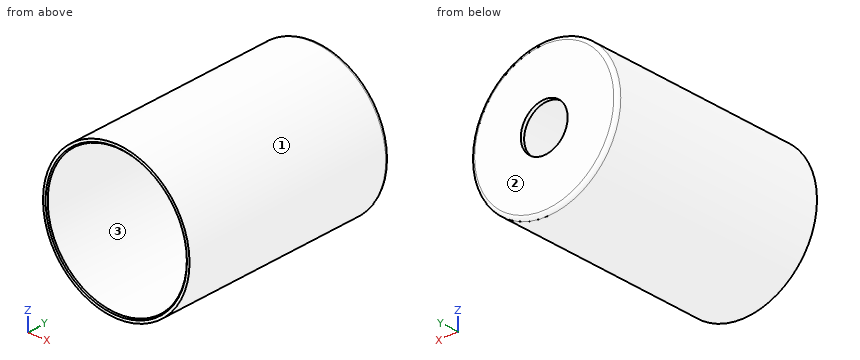
```python
from build123d import *

# Parameters (mm, degrees)
F0_R          = 50.8
F1_DEPTH      = 152.4
F2_T          = -2.54
F3_R          = 16.25
F4_DEPTH      = 25.4
F4_DEPTH_BACK = 25.4
F5_SIZE       = 0.762
F6_R          = 2.54


with BuildPart() as f1:
    # F0 (on Front) → F1 (new body)
    with BuildSketch(Plane.XZ):
        Circle(F0_R)
    extrude(amount=F1_DEPTH)

    # F2
    f2_openings = [f1.faces().sort_by_distance(p)[0] for p in [
        (0, -152.4, 0),
    ]]
    offset(amount=F2_T, openings=f2_openings)

    # F3 (on face) → F4 (cut, two sides)
    with BuildSketch(Plane.XZ.offset(2.54)) as f4_sk:
        Circle(F3_R)
    extrude(amount=-F4_DEPTH, mode=Mode.SUBTRACT)
    extrude(f4_sk.sketch, amount=F4_DEPTH_BACK, mode=Mode.SUBTRACT)

    # F5
    f5_edges = [f1.edges().sort_by_distance(p)[0] for p in [
        (-48.26, -152.4, 0),
    ]]
    chamfer(f5_edges, length=F5_SIZE)

    # F6
    f6_edges = [f1.edges().sort_by_distance(p)[0] for p in [
        (-50.8, 0, 0),
    ]]
    fillet(f6_edges, radius=F6_R)


solid = f1.part
```
Here's how the part is built. I have some questions about the finished solid (model axes, mm). Face numbers are marked on the shaded views. Give positions to 0.01 mm unless a question says otherwise; leave off trailing zeros. Loops run counter-clockwise (first coordinate to the right, second up) from the corner with the lowest first, then second, coordinate; pieces in that order, holes last. Notation, with made-up numbers: M 61.25,4 L 101.25,4 A5 cw 101.25,8 Z; hole C -5.5,82.5 d4. An arc over 180 degrees is marked long. Put each result on its own line as item: value. Start each with the question number.
(1) I want a section at C-C on y = -24.5. Please give me the cut outline in (x, z).
(2) If we mould it in two halves opening along Z, with no side actions, what happens to the marked faces 1, 2 and 3? For each: +Z half, -Z half, draft (parallel to the pull), parting line (faces both ways), or undercut.
(3) Will these pins go through, and if not, where does the flat tip stop? pin 1 Ø12 at (y, z) = (-132, -16.5) entering from -X; pin 2 Ø1 at (y, z) = (-116.5, -21) entering from +X; pin 3 Ø1.5 at (y, z) = (-82, -16.5) entering from -X.
(4) I need wall thicknesses on line 1 along Z through (x, y) = (-20.5, -47.5); line 2 along Z through (x, y) = (-19.5, -91); line 3 along X through (y, z) = (-63, -22). Which ranges of each line are inside material? Lowest first, please. Write a range as [from, to].
(5) I want a section at A-A on z = 0. Please give me the cut outline in (x, y).
(6) I want a section at B-B on x = 0. Please give me the cut outline in (y, z), then the cut area to 3 significant figures.
Answer block:
1. outline: C 0,0 d101.6; hole C 0,0 d96.52
2. face 1: parting line
2. face 2: draft
2. face 3: undercut
3. pin 1: x = -49.7
3. pin 2: x = 46.48
3. pin 3: x = -48.3
4. line 1: [-46.48, -43.69], [43.69, 46.48]
4. line 2: [-46.91, -44.14], [44.14, 46.91]
4. line 3: [-45.79, -42.95], [42.95, 45.79]
5. outline: M -50.8,-152.4 L -49.02,-152.4 L -48.26,-151.64 L -48.26,-2.54 L -16.25,-2.54 L -16.25,0 L -48.26,0 A2.54 ccw -50.8,-2.54 Z; M 16.25,-2.54 L 48.26,-2.54 L 48.26,-151.64 L 49.02,-152.4 L 50.8,-152.4 L 50.8,-2.54 A2.54 ccw 48.26,0 L 16.25,0 Z
6. outline: M -152.4,-50.8 L -2.54,-50.8 A2.54 ccw 0,-48.26 L 0,-16.25 L -2.54,-16.25 L -2.54,-48.26 L -151.64,-48.26 L -152.4,-49.02 Z; M -152.4,49.02 L -151.64,48.26 L -2.54,48.26 L -2.54,16.25 L 0,16.25 L 0,48.26 A2.54 ccw -2.54,50.8 L -152.4,50.8 Z
6. area: 933 mm^2
